from build123d import *

# Parameters (mm, degrees)
SKETCH1_W          = 260
SKETCH1_H          = 185
EXTRUDE1_DEPTH     = 3
FILLET3_R          = 6
SKETCH2_W          = 40
SKETCH2_H          = 25
CUT_EXTRUDE1_DEPTH = 320.11439955
FILLET1_R          = 2
FILLET2_R          = 1


with BuildPart() as part:
    # Sketch1 → Extrude1 (new body)
    with BuildSketch(Plane(origin=(0, 0, 0), x_dir=(1, 0, 0), z_dir=(0, 1, 0))):
        with Locations((130, 92.5)):
            Rectangle(SKETCH1_W, SKETCH1_H)
    extrude(amount=EXTRUDE1_DEPTH)

    # Fillet3
    fillet3_edges = [part.edges().sort_by_distance(p)[0] for p in [
        (0, 1.5, -185),
        (260, 1.5, -185),
        (260, 1.5, 0),
        (0, 1.5, 0),
    ]]
    fillet(fillet3_edges, radius=FILLET3_R)

    # Sketch2 → Cut-Extrude1 (cut, through all)
    with BuildSketch(Plane(origin=(0, 3, 0), x_dir=(-1, 0, 0), z_dir=(0, 1, 0))):
        with Locations((-30, -22.5)):
            Rectangle(SKETCH2_W, SKETCH2_H)
    extrude(amount=-CUT_EXTRUDE1_DEPTH, mode=Mode.SUBTRACT)

    # Fillet1
    fillet1_edges = [part.edges().sort_by_distance(p)[0] for p in [
        (10, 1.5, -10),
        (10, 1.5, -35),
        (50, 1.5, -35),
        (50, 1.5, -10),
    ]]
    fillet(fillet1_edges, radius=FILLET1_R)

    # Fillet2
    fillet2_edges = [part.edges().sort_by_distance(p)[0] for p in [
        (30, 3, -35),
        (50, 3, -22.5),
        (30, 3, -10),
        (10, 3, -22.5),
        (49.414213562, 3, -34.414213562),
        (49.414213562, 3, -10.585786438),
        (10.585786438, 3, -10.585786438),
        (10.585786438, 3, -34.414213562),
    ]]
    fillet(fillet2_edges, radius=FILLET2_R)


solid = part.part
Read the model definition and answer for the solid it produces. Units are mm, in the model's axes. Coordinates: 2 decimals unless noted, no trailing zeros. Order: outer loops, then holes, each group sorted by start corner. A loop starts at its lowest first (then second) coordinate and runs counter-clockwise, first axis right, second up. Notation, with made-up numbers: M 45,-10 L 85,-10 A25 cw 85,14 Z; hole C 60.5,64 d5. An arc over 180 degrees is marked long. Put each result on its own line as item: value. Start each with the question number.
Item 1: Section A-A, the plane z = -25 is taken. Determine the outline of the cut face in (x, y), plus the area to 3 significant figures.
Item 2: Given pin 1 Ø8 at (x, z) = (56.5, -100) entering from -Y, flat-ended and moving along its own axis, determine where the tip first touches the part or whether it passes through.
Item 3: Consider probe 1 along Z at (x, y) = (27.5, 2.25); probe 2 along Z at (x, y) = (48.5, 1); probe 3 along X at (y, z) = (0.6, -33). Determine where each line is inside the solid, lowest interval first. Write a range as [from, to].
Item 4: Section B-B, the plane y = 0.45 is taken. Determine the outline of the cut face in (x, z), plus the area to 3 significant figures.
Computed:
1. outline: M 0,0 L 10,0 L 10,2 A1 ccw 9,3 L 0,3 Z; M 50,0 L 260,0 L 260,3 L 51,3 A1 ccw 50,2 Z
1. area: 660 mm2
2. pin 1: stops at y = 0
3. probe 1: z = [-185, -35.03], [-9.97, 0]
3. probe 2: z = [-185, -34.94], [-10.06, 0]
3. probe 3: x = [0, 10], [50, 260]
4. outline: M 0,-179 A6 ccw 6,-185 L 254,-185 A6 ccw 260,-179 L 260,-6 A6 ccw 254,0 L 6,0 A6 ccw 0,-6 Z; hole M 10,-33 A2 ccw 12,-35 L 48,-35 A2 ccw 50,-33 L 50,-12 A2 ccw 48,-10 L 12,-10 A2 ccw 10,-12 Z
4. area: 47,100 mm2
